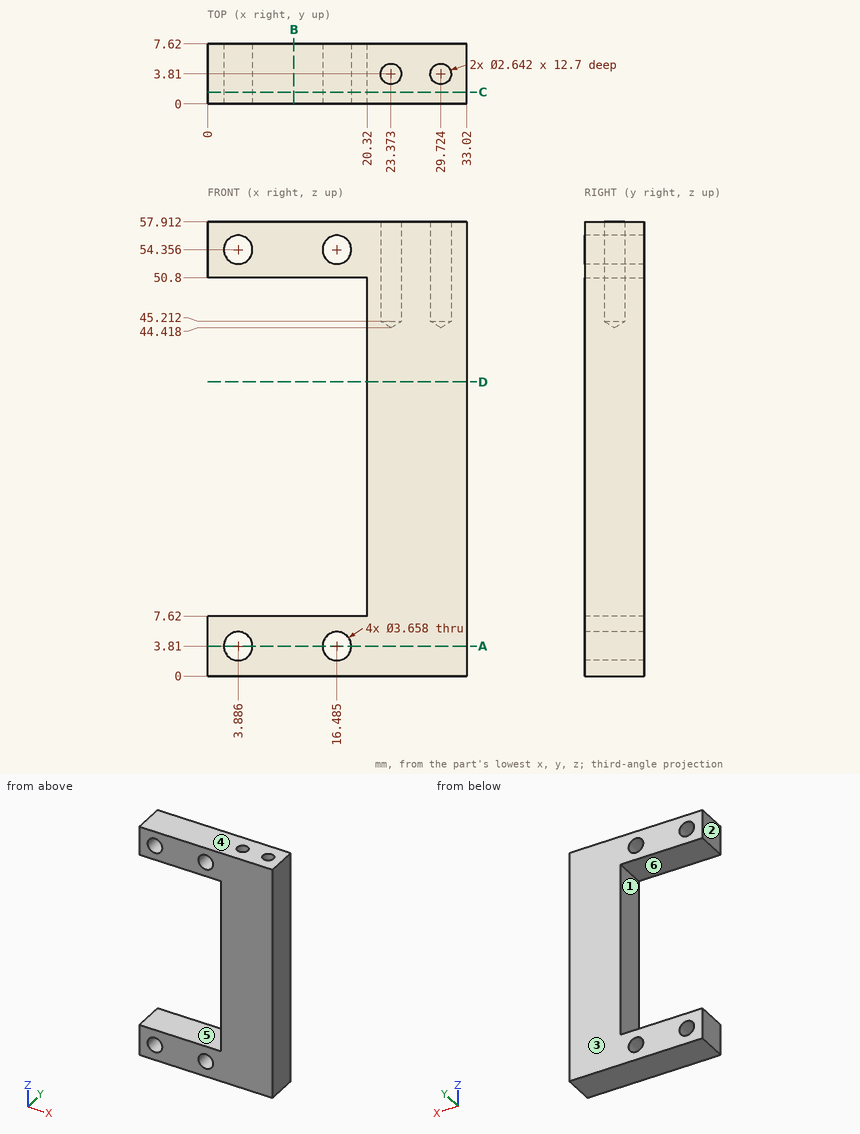
Study the drawing (mm; zero at the part's minimum x, y, z) and answer. A direction names the side the tool comes from. Round coordinates to 2 decimals unless told otherwise and drop trailing zeros. Order: outer loops, then holes, each group sorted by start corner. A loop starts at its lowest first (then second) coordinate and runs counter-clockwise, first axis right, second up. Notation, with made-up numbers: M 74,-30.5 L 109,-30.5 A14 cw 109,-3.5 Z; hole C 67.5,0.5 d7. An arc over 180 degrees is marked long. One line per item, written item: value.
Q1. Find section D-D on z = 37.5. Write down the section's boundary in (x, y).
Derived:
outline: M 20.32,0 L 33.02,0 L 33.02,7.62 L 20.32,7.62 Z
Q2. For the marked faces 1 and 2, determine the directions among +Z, -Z, +X, -X, +Y, -Y from which every point of the face is accessible in a straight line to the end or side of a thin tool.
Derived:
face 1: -X, +Y, -Y
face 2: +Z, -Z, -X, +Y, -Y
Q3. Straight lines are drawn through the part: line 1 (X direction, y = 4, z = 51); line 2 (X direction, y = 3.81, z = 48.25) (1 decimal); line 3 (Z direction, x = 13.5, y = 2). For each, find the intervals that lie inside material, in ascending order.
Derived:
line 1: 0 to 22.07, 24.68 to 28.42, 31.03 to 33.02
line 2: 20.3 to 22.1, 24.7 to 28.4, 31 to 33
line 3: 0 to 7.62, 50.8 to 57.91
Q4. Find section A-A on z = 3.81. Write down the section's boundary in (x, y) (1 decimal), then the cut area to 3 significant figures.
Derived:
outline: M 0,0 L 2.1,0 L 2.1,7.6 L 0,7.6 Z; M 5.7,0 L 14.7,0 L 14.7,7.6 L 5.7,7.6 Z; M 18.3,0 L 33,0 L 33,7.6 L 18.3,7.6 Z
area: 196 mm²
Q5. Find section B-B on x = 11. Write down the section's boundary in (y, z).
Derived:
outline: M 0,0 L 7.62,0 L 7.62,7.62 L 0,7.62 Z; M 0,50.8 L 7.62,50.8 L 7.62,57.91 L 0,57.91 Z
Q6. Find section C-C on y = 1.5. Write down the section's boundary in (x, z) (1 decimal).
Derived:
outline: M 0,0 L 33,0 L 33,57.9 L 0,57.9 L 0,50.8 L 20.3,50.8 L 20.3,7.6 L 0,7.6 Z; hole C 3.9,3.8 d3.7; hole C 3.9,54.4 d3.7; hole C 16.5,3.8 d3.7; hole C 16.5,54.4 d3.7
Q7. Determine the mould class of the marked faces 3, 4, 5 and 6 for opening direction Z: released by +Z, released by -Z, zero draft, split by the parting line, or undercut.
Derived:
face 3: zero draft
face 4: released by +Z
face 5: undercut
face 6: undercut
Q8. Flat-ended cylindrical pins translate along their axes: pin 1 (2.5 mm diameter, centred on y = 2.5, z = 37.5, fed in from -X); pin 2 (2.5 mm diameter, centred on x = 23.37, y = 3.81, fed in from +Z). Find the tip coordinate at first contact, or state that the pin passes through.
Derived:
pin 1: x = 20.32
pin 2: z = 45.17
